from build123d import *

# Parameters (mm, degrees)
SKETCH1_R           = 1.1
BOSS_EXTRUDE1_DEPTH = 4.7625
FILLET1_R           = 5
SKETCH3_R           = 5.1
CUT_EXTRUDE2_DEPTH  = 5.7625


with BuildPart() as part:
    # Sketch1 → Boss-Extrude1 (new body)
    with BuildSketch(Plane.XY):
        with BuildLine():
            Line((-30.671332299, 7.5), (-26.768089678, 10))
            ThreePointArc((-26.768089678, 10), (0, 28.575), (26.768089678, 10))
            Line((26.768089678, 10), (30.671332299, 7.5))
            ThreePointArc((30.671332299, 7.5), (31.575, 0), (30.671332299, -7.5))
            Line((30.671332299, -7.5), (26.768089678, -10))
            ThreePointArc((26.768089678, -10), (0, -28.575), (-26.768089678, -10))
            Line((-26.768089678, -10), (-30.671332299, -7.5))
            ThreePointArc((-30.671332299, -7.5), (-31.575, 0), (-30.671332299, 7.5))
        make_face()
        with Locations((-25.4, 0)):
            Circle(SKETCH1_R, mode=Mode.SUBTRACT)
        with Locations((-12.7, 21.997045256)):
            Circle(SKETCH1_R, mode=Mode.SUBTRACT)
        with Locations((12.7, 21.997045256)):
            Circle(SKETCH1_R, mode=Mode.SUBTRACT)
        with Locations((25.4, 0)):
            Circle(SKETCH1_R, mode=Mode.SUBTRACT)
        with Locations((12.7, -21.997045256)):
            Circle(SKETCH1_R, mode=Mode.SUBTRACT)
        with Locations((-12.7, -21.997045256)):
            Circle(SKETCH1_R, mode=Mode.SUBTRACT)
    extrude(amount=BOSS_EXTRUDE1_DEPTH)

    # Fillet1
    fillet1_edges = [part.edges().sort_by_distance(p)[0] for p in [
        (30.671332299, -7.5, 2.38125),
        (26.768089678, -10, 2.38125),
        (-26.768089678, -10, 2.38125),
        (-30.671332299, -7.5, 2.38125),
        (-30.671332299, 7.5, 2.38125),
        (-26.768089678, 10, 2.38125),
        (26.768089678, 10, 2.38125),
        (30.671332299, 7.5, 2.38125),
    ]]
    fillet(fillet1_edges, radius=FILLET1_R)

    # Sketch3 → Cut-Extrude2 (cut, through all)
    with BuildSketch(Plane.XY.offset(4.7625)):
        with Locations((0, -9.25)):
            Circle(SKETCH3_R)
        with Locations((0, 9.25)):
            Circle(SKETCH3_R)
    extrude(amount=-CUT_EXTRUDE2_DEPTH, mode=Mode.SUBTRACT)


solid = part.part
Geometry: final body of the model. Coordinates: model frame, mm. Give positions to 0.01 mm unless a question says otherwise; leave off trailing zeros. Loops run counter-clockwise (first coordinate to the right, second up) from the corner with the lowest first, then second, coordinate; pieces in that order, holes last. Notation, with made-up numbers: (71, -8) - (89, -8) arc R24 ccw to (89, 8) - close; hole circle Ø7 at (-3.75, 63.25). An arc over 180 degrees is marked (long way). One line per question, with ' | ' between items. Start each with the question number.
(1) Section query D-D on y = 10. Return loops of the section in (x, z), then the cut area to 3 significant figures.
(2) Pull-direction query (Y, two-part tool) for faces 1 (the cylindrical face through (26.45, 0.33, 2.35)), 2 (the cylindrical face through (-30.39, -7.16, 2.41)), 3 (the cylindrical face through (-0.46, 28.57, 2.35)); classes: released by +Y, released by -Y, zero draft, split by the parting line, or undercut.
(3) Section query A-A on y = 0. Return loops of the section in (x, z) (1 decimal), then the cut area to 3 significant figures.
(4) Section query B-B on x = 0. Count the separate pieces of the cut face and the enclosed holes in it, then the cut area to 3 significant figures.
(5) Ray query, line 1 (Y direction, x = 4, z = 1.05); line 2 (Y direction, x = -2.5, z = 1.4); line 3 (X direction, y = -23, z = 1.85). Return the intervals inside material, ascending. Write a range as from..to.
(6) Section query C-C on x = -25.4. Return loops of the section in (y, z), then the cut area to 3 significant figures.
(7) Contact query for flat-ended pins moving along their axis: pin 1 (1.3 mm diameter, centred on x = 25.4, y = 0, fed in from -Z); pin 2 (1.5 mm diameter, centred on y = 1, z = 1, fed in from -X); pin 3 (2 mm diameter, centred on x = -2.5, z = 3.5, fed in from -Y). Output: stop coordinate, or through.
The answers:
1) outline: (-27.1, 0) - (-5.04, 0) - (-5.04, 4.76) - (-27.1, 4.76) - close; (5.04, 0) - (27.1, 0) - (27.1, 4.76) - (5.04, 4.76) - close | area: 210 mm2
2) face 1: undercut | face 2: released by -Y | face 3: released by +Y
3) outline: (-31.6, 0) - (-26.5, 0) - (-26.5, 4.8) - (-31.6, 4.8) - close; (-24.3, 0) - (24.3, 0) - (24.3, 4.8) - (-24.3, 4.8) - close; (26.5, 0) - (31.6, 0) - (31.6, 4.8) - (26.5, 4.8) - close | area: 280 mm2
4) separate pieces: 3 | enclosed holes: 0 | area: 175 mm2
5) line 1: -28.29..-12.41, -6.09..6.09, 12.41..28.29 | line 2: -28.47..-13.7, -4.8..4.8, 13.7..28.47 | line 3: -16.96..-13.15, -12.25..12.25, 13.15..16.96
6) outline: (-13.09, 0) - (-1.1, 0) - (-1.1, 4.76) - (-13.09, 4.76) - close; (1.1, 0) - (13.09, 0) - (13.09, 4.76) - (1.1, 4.76) - close | area: 114 mm2
7) pin 1: through | pin 2: x = -31.57 | pin 3: y = -28.54
